from build123d import *

# Parameters (mm, degrees)
SKETCH1_W           = 135
SKETCH1_H           = 135
BOSS_EXTRUDE1_DEPTH = 45
SKETCH2_R           = 10
SKETCH2_R_2         = 30
CUT_EXTRUDE1_DEPTH  = 106.534354596
SKETCH3_R           = 55.5
CUT_EXTRUDE2_DEPTH  = 30
SKETCH4_R           = 35
CUT_EXTRUDE3_DEPTH  = 10


with BuildPart() as part:
    # Sketch1 → Boss-Extrude1 (new body)
    with BuildSketch(Plane.XY):
        Rectangle(SKETCH1_W, SKETCH1_H)
    extrude(amount=BOSS_EXTRUDE1_DEPTH)

    # Sketch2 → Cut-Extrude1 (cut, through all)
    with BuildSketch(Plane.XY.offset(45)):
        with Locations((-47.5, 47.5)):
            Circle(SKETCH2_R)
        with Locations((47.5, 47.5)):
            Circle(SKETCH2_R)
        with Locations((47.5, -47.5)):
            Circle(SKETCH2_R)
        with Locations((-47.5, -47.5)):
            Circle(SKETCH2_R)
        Circle(SKETCH2_R_2)
    extrude(amount=-CUT_EXTRUDE1_DEPTH, mode=Mode.SUBTRACT)

    # Sketch3 → Cut-Extrude2 (cut)
    with BuildSketch(Plane.XY.offset(45)):
        Circle(SKETCH3_R)
    extrude(amount=-CUT_EXTRUDE2_DEPTH, mode=Mode.SUBTRACT)

    # Sketch4 → Cut-Extrude3 (cut)
    with BuildSketch(Plane.XY.offset(15)):
        Circle(SKETCH4_R)
    extrude(amount=-CUT_EXTRUDE3_DEPTH, mode=Mode.SUBTRACT)


solid = part.part
CAD build for the part. Positions are in the model's coordinates, mm. A direction names the side the tool comes from. Coordinates: 2 decimals unless noted, no trailing zeros. Order: outer loops, then holes, each group sorted by start corner. A loop starts at its lowest first (then second) coordinate and runs counter-clockwise, first axis right, second up. Notation, with made-up numbers: (52, 72.5) -> (82, 72.5) arc R17 cw to (82, 93.5) -> close; hole circle Ø10 at (2.5, 7). An arc over 180 degrees is marked (long way). Answer in a Markdown table with one row per item.
1) Flat gauge pin, fed straight in: P1, Ø18, axis at x = 47.5, y = -47.5, coming from the -Z side. Where does the tip first touch, or does it go through?
Check values:
| item | result |
|---|---|
| P1 | through |
2) Drill centre lines: line 1 (Y direction, x = -47.5, z = 10.5); line 2 (Y direction, x = 0, z = 22.75); line 3 (Y direction, x = 0, z = 11.5). Where is each one in solid material? Low to high.
Check values:
| item | result |
|---|---|
| line 1 | -67.5 to -57.5, -37.5 to 37.5, 57.5 to 67.5 |
| line 2 | -67.5 to -55.5, 55.5 to 67.5 |
| line 3 | -67.5 to -35, 35 to 67.5 |
3) Band-saw the part on D-D (x = 47.5). List the corners of the cut face in (y, z), and give its area (3 significant figures).
Check values:
| item | result |
|---|---|
| outline | (-67.5, 0) -> (-57.5, 0) -> (-57.5, 45) -> (-67.5, 45) -> close; (-37.5, 0) -> (37.5, 0) -> (37.5, 45) -> (28.71, 45) -> (28.71, 15) -> (-28.71, 15) -> (-28.71, 45) -> (-37.5, 45) -> close; (57.5, 0) -> (67.5, 0) -> (67.5, 45) -> (57.5, 45) -> close |
| area | 2,550 mm2 |
4) Band-saw the part on A-A (z = 7). List the corners of the cut face in (x, y), and give its area (3 significant figures).
Check values:
| item | result |
|---|---|
| outline | (-67.5, -67.5) -> (67.5, -67.5) -> (67.5, 67.5) -> (-67.5, 67.5) -> close; hole circle Ø20 at (-47.5, -47.5); hole circle Ø20 at (-47.5, 47.5); hole circle Ø70 at (0, 0); hole circle Ø20 at (47.5, -47.5); hole circle Ø20 at (47.5, 47.5) |
| area | 13,100 mm2 |
5) Mould opens along Y. For faces 1 (the face through (-1, 67.5, 22)), 2 (the face through (-1, 31, 0)), 3 (the face through (-55.44, -53.58, 22.82)) say: pulls with the +Y half, pulls with the -Y half, needs draft (parallel to the pull), parting line crosses it, or undercut.
Check values:
| item | result |
|---|---|
| face 1 | pulls with the +Y half |
| face 2 | needs draft |
| face 3 | undercut |
6) Which spindle directions (+Z, -Z, +X, -X, +Y, -Y) get a long thin tool onto all of the face, cutting with end or side? Do faces 4 (the face through (-28, -21, 10)), 5 (the face through (67.5, -1, 22)). Say none if no direction does.
Check values:
| item | result |
|---|---|
| face 4 | +Z |
| face 5 | +Z, -Z, +X, +Y, -Y |
7) Band-saw the part on B-B (x = 0). List the corners of the cut face in (y, z).
Check values:
| item | result |
|---|---|
| outline | (-67.5, 0) -> (-30, 0) -> (-30, 5) -> (-35, 5) -> (-35, 15) -> (-55.5, 15) -> (-55.5, 45) -> (-67.5, 45) -> close; (30, 0) -> (67.5, 0) -> (67.5, 45) -> (55.5, 45) -> (55.5, 15) -> (35, 15) -> (35, 5) -> (30, 5) -> close |
